Model file for the job. Use its own axes, mm. Face numbers are marked on the shaded views. A direction names the side the tool comes from. Give positions to 0.01 mm unless a question says otherwise; leave off trailing zeros. Loops run counter-clockwise (first coordinate to the right, second up) from the corner with the lowest first, then second, coordinate; pieces in that order, holes last. Notation, with made-up numbers: (80.25, -13) - (108.25, -13) arc R20 cw to (108.25, 1) - close; hole circle Ø4 at (-19, 57). An arc over 180 degrees is marked (long way). Answer as CSV lines item,"result". Start each with the question number.
Item 1: Tool access for the marked faces 4, 5 and 6: list every direction of +Z, -Z, +X, -X, +Y, -Y with a clear straight run to the whole face (end or side of a thin tool).
Item 2: Saw through at C-C on z = 3.5. Give the cut face in (x, y).
Item 3: Pin check, flat tips, straight feed: pin 1 (10 mm diameter, centred on x = 12.7, y = 0, fed in from -Z); pin 2 (6.5 mm diameter, centred on y = -3, z = 23.5, fed in from -X); pin 3 (5 mm diameter, centred on x = 24.5, y = -6, fed in from +Z); pin 4 (7.5 mm diameter, centred on x = 116.5, y = 7, fed in from +Z). Stop position of each tip, or through.
Item 4: Saw through at D-D on y = -1.5. Give the cut face in (x, z), plus the area to 3 significant figures.
Item 5: Drill centre lines: L1, parallel to Y at x = 12.7, z = 11; L2, parallel to Z at x = 10, y = 17.5; L3, parallel to Y at x = 113, z = 18. Where is each one in solid material? Low to high. Write a range as from..to.
Item 6: Pull direction X, two halves, no side cores. Call the marked faces 1, 2 and 3: pulls with the +X half, pulls with the -X half, needs draft (parallel to the pull), parting line crosses it, or undercut.
Item 7: Saw through at A-A on x = 114.3. Give the cut face in (y, z).
Item 8: Saw through at B-B on y = 13.5. Give the cut face in (x, z), plus the area to 3 significant figures.
from build123d import *

# Parameters (mm, degrees)
F1_DEPTH = 19.05
F3_D     = 12.7
F3_DEPTH = 31.75
F6_DEPTH = 12.7


with BuildPart() as f1:
    # F0 (on Front) → F1 (new body, symmetric)
    with BuildSketch(Plane.XZ):
        Polygon((0, 25.4), (0, 0), (127, 0), (127, 25.4), (101.6, 25.4), (88.9, 50.8), (38.1, 50.8), (25.4, 25.4), align=None)
    extrude(amount=F1_DEPTH, both=True)

    # F3
    with Locations(Plane.XY.offset(25.4)):
        with Locations((12.7, 0), (114.3, 0)):
            Hole(F3_D / 2, depth=F3_DEPTH)

    # F5 (on offset) → F6 (cut, symmetric)
    with BuildSketch(Plane.YZ.offset(63.5)):
        Polygon((-19.05, 12.7), (2.947045, 50.8), (-19.05, 50.8), align=None)
    extrude(amount=F6_DEPTH, both=True, mode=Mode.SUBTRACT)


solid = f1.part
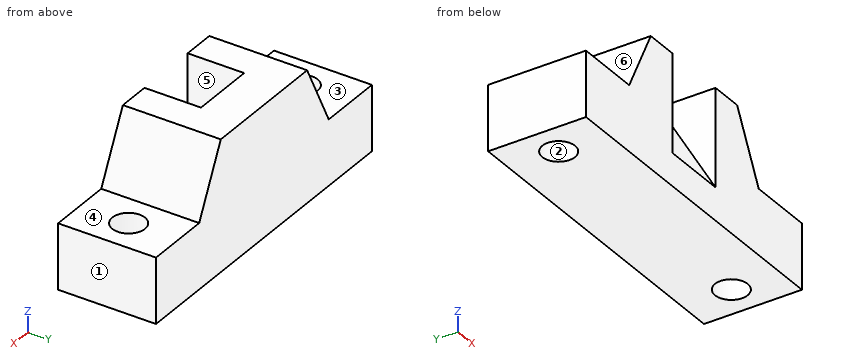
Responses:
1,face 4,"+Z, +X, +Y, -Y"
1,face 5,"+Z, -Y"
1,face 6,"+Z, -X, +Y, -Y"
2,outline,"(0, -19.05) - (127, -19.05) - (127, 19.05) - (0, 19.05) - close; hole circle Ø12.7 at (12.7, 0); hole circle Ø12.7 at (114.3, 0)"
3,pin 1,"through"
3,pin 2,"x = 0"
3,pin 3,"z = 28.6"
3,pin 4,"z = 25.4"
4,outline,"(0, 0) - (6.53, 0) - (6.53, 25.4) - (0, 25.4) - close; (18.87, 0) - (108.13, 0) - (108.13, 25.4) - (101.6, 25.4) - (88.9, 50.8) - (76.2, 50.8) - (76.2, 43.1) - (50.8, 43.1) - (50.8, 50.8) - (38.1, 50.8) - (25.4, 25.4) - (18.87, 25.4) - close; (120.47, 0) - (127, 0) - (127, 25.4) - (120.47, 25.4) - close"
4,area,"4,020 mm2"
5,L1,"-19.05..-6.35, 6.35..19.05"
5,L2,"0..25.4"
5,L3,"-19.05..-6.22, 6.22..19.05"
6,face 1,"pulls with the +X half"
6,face 2,"undercut"
6,face 3,"needs draft"
7,outline,"(-19.05, 0) - (-6.35, 0) - (-6.35, 25.4) - (-19.05, 25.4) - close; (6.35, 0) - (19.05, 0) - (19.05, 25.4) - (6.35, 25.4) - close"
8,outline,"(0, 0) - (127, 0) - (127, 25.4) - (101.6, 25.4) - (88.9, 50.8) - (38.1, 50.8) - (25.4, 25.4) - (0, 25.4) - close"
8,area,"4,840 mm2"
